Design review of the part built by this model. Coordinates are the model's own, in mm. Face numbers are marked on the shaded views. Coordinates: 2 decimals unless noted, no trailing zeros. Order: outer loops, then holes, each group sorted by start corner. A loop starts at its lowest first (then second) coordinate and runs counter-clockwise, first axis right, second up. Notation, with made-up numbers: M 44.5,-3.75 L 68.5,-3.75 A14 ccw 68.5,21.25 Z; hole C 65,49.5 d4. An arc over 180 degrees is marked long. Answer as a JSON object with one key per item and string values.
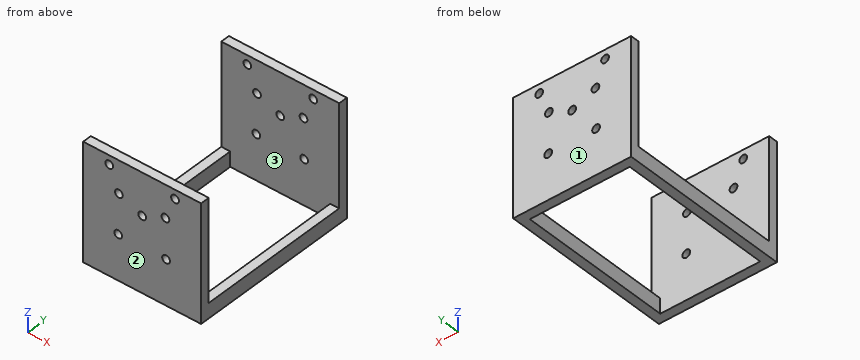
Autodesk Inventor part; units mm, degrees
ref_plane "YZ Plane" through (0, 0, 0) normal (1, 0, 0) x (0, 1, 0)
ref_plane "XZ Plane" through (0, 0, 0) normal (0, 1, 0) x (-1, 0, 0)
ref_plane "XY Plane" through (0, 0, 0) normal (0, 0, 1) x (1, 0, 0)
sketch "스케치1" plane through (0, 0, 0) normal (0, 0, 1) x (1, 0, 0)
  line L0 (-16.7, 25.65) -> (16.7, 25.65)
  line L1 (16.7, 25.65) -> (16.7, -25.65)
  line L2 (16.7, -25.65) -> (-16.7, -25.65)
  line L3 (-16.7, -25.65) -> (-16.7, 25.65)
  line L4 (19.7, 28.65) -> (-19.7, 28.65)
  line L5 (-19.7, 28.65) -> (-19.7, -28.65)
  line L6 (-19.7, -28.65) -> (19.7, -28.65)
  line L7 (19.7, -28.65) -> (19.7, 28.65)
  point P0 (0, 0)
  point P1 (-16.7, 0)
  point P2 (0, 25.65)
  dimension "d0" = 33.4
  dimension "d1" = 51.3
  dimension "d2" = 3
extrude "돌출1" add sketch "스케치1" along normal blind 5
sketch "스케치5" plane through (-19.7, -28.65, 0) normal (0, -1, 0) x (1, 0, 0)
  line L0 (0, 0) -> (39.4, 0)
  line L1 (39.4, 0) -> (39.4, 5)
  line L2 (0, 5) -> (39.4, 5)
  line L3 (0, 0) -> (0, 5)
  circle A0 centre (8.7, 36) radius 1.3
  circle A1 centre (11.9218, 28.2218) radius 1.3
  circle A2 centre (19.7, 25) radius 1.3
  circle A3 centre (27.4782, 28.2218) radius 1.3
  circle A4 centre (30.7, 36) radius 1.3
  line L4 (0, 0) -> (39.4, 0)
  line L5 (39.4, 0) -> (39.4, 39)
  line L6 (39.4, 39) -> (0, 39)
  line L7 (0, 39) -> (0, 0)
  line L8 (0, 15) -> (39.4, 15) construction
  line L9 (19.7, 39) -> (19.7, 5) construction
  circle A5 centre (11.7, 15) radius 1.3
  circle A6 centre (27.7, 15) radius 1.3
  point P0 (19.7, 36)
  dimension "d46" = 180
  dimension "d52" = 39
  dimension "d53" = 24
  dimension "d54" = 2.6
  dimension "d55" = 8
extrude "돌출2" add sketch "스케치5" against normal blind 3 contours L7 L6 L5 L2
mirror "미러1" about plane through (0, 0, 0) normal (0, 1, 0)
properties part number "MX64 FRAME"
1) Add section C-C (y = -10.5). State the section outline as (x, z) points.
Taken from the geometry:
{"outline": "M -19.7,0 L -16.7,0 L -16.7,5 L -19.7,5 Z; M 16.7,0 L 19.7,0 L 19.7,5 L 16.7,5 Z"}
2) To check wall thickness, follow L1, parallel to Y at x = 10, z = 12.5; L2, parallel to Z at x = -11, y = 27; L3, parallel to Z at x = 8, y = -27.35. State the ranges of each line that lie inside material, in increasing order.
Taken from the geometry:
{"L1": "y = -28.65 to -25.65, 25.65 to 28.65", "L2": "z = 0 to 34.7, 37.3 to 39", "L3": "z = 0 to 13.7, 16.3 to 26.94, 29.5 to 39"}
3) Add section B-B (x = 0). State the section outline as (y, z) points.
Taken from the geometry:
{"outline": "M -28.65,0 L -25.65,0 L -25.65,23.7 L -28.65,23.7 Z; M -28.65,26.3 L -25.65,26.3 L -25.65,39 L -28.65,39 Z; M 25.65,0 L 28.65,0 L 28.65,23.7 L 25.65,23.7 Z; M 25.65,26.3 L 28.65,26.3 L 28.65,39 L 25.65,39 Z"}
4) Add section D-D (z = 15). State the section outline as (x, y) points, and give its area (3 significant figures).
Taken from the geometry:
{"outline": "M -19.7,-28.65 L -9.3,-28.65 L -9.3,-25.65 L -19.7,-25.65 Z; M -19.7,25.65 L -9.3,25.65 L -9.3,28.65 L -19.7,28.65 Z; M -6.7,-28.65 L 6.7,-28.65 L 6.7,-25.65 L -6.7,-25.65 Z; M -6.7,25.65 L 6.7,25.65 L 6.7,28.65 L -6.7,28.65 Z; M 9.3,-28.65 L 19.7,-28.65 L 19.7,-25.65 L 9.3,-25.65 Z; M 9.3,25.65 L 19.7,25.65 L 19.7,28.65 L 9.3,28.65 Z", "area": "205 mm2"}
5) Insertion check: pin 1 Ø4 at (x, y) = (-13, 4.5) entering from -Z; pin 2 Ø1.5 at (x, y) = (-18, -3.5) entering from +Z. Each pin has a flat end and moves straight along its axis. Give the tip position at first contact, or say it passes through.
Taken from the geometry:
{"pin 1": "passes through", "pin 2": "stops at z = 5"}
6) Add section A-A (z = 22.5). State the section outline as (x, y) points.
Taken from the geometry:
{"outline": "M -19.7,-28.65 L 19.7,-28.65 L 19.7,-25.65 L -19.7,-25.65 Z; M -19.7,25.65 L 19.7,25.65 L 19.7,28.65 L -19.7,28.65 Z"}
7) Mouldability with a two-part tool opening along Y and no side actions: class the marked faces 1, 2 and 3 as released by +Y, released by -Y, zero draft, split by the parting line, or undercut.
Taken from the geometry:
{"face 1": "released by +Y", "face 2": "released by -Y", "face 3": "undercut"}
